The listing builds one solid part. Answer for the finished solid, in the listing's coordinates (mm). Face numbers are marked on the shaded views. Give positions to 0.01 mm unless a question says otherwise; leave off trailing zeros. Write each loop counter-clockwise with the first axis right and the second up, starting at its lowest first coordinate (ties: lowest second). Pieces come first, ordered by that corner, then holes. Notation, with made-up numbers: (53.25, 28) - (74.25, 28) arc R36 cw to (74.25, 67) - close; hole circle Ø1 at (74, 71). An arc over 180 degrees is marked (long way). Answer as CSV lines item,"result". Start each with the question number.
(1) Find section D-D (y = -4.25). Write down the section's boundary in (x, z).
(2) Straight lines are drawn through the part: probe 1 along Y at (x, z) = (3.25, 12); probe 2 along Y at (x, z) = (3.25, 37); probe 3 along Y at (x, z) = (19.75, 35.5). For each, find the intervals that lie inside material, in ascending order.
(3) Find section B-B (z = 38.5). Write down the section's boundary in (x, y).
(4) Each of these flat-tipped pins is pushed along its axis until it touches: pin 1 Ø3 at (x, z) = (19, 37.5) entering from -Y; pin 2 Ø3 at (x, y) = (8.5, -3) entering from -Z; pin 3 Ø8 at (x, z) = (9, 4) entering from -Y. Where does it stop, or does it pass through?
(5) For a pull along Y with two mould halves and no side action, classify the marked faces 1, 2 and 3 as pulls with the +Y half, pulls with the -Y half, needs draft (parallel to the pull), parting line crosses it, or undercut.
(6) Find section C-C (z = 9). Write down the section's boundary in (x, y), then the cut area to 3 significant figures.
from build123d import *

# Parameters (mm, degrees)
F0_W     = 27
F0_H     = 43
F1_DEPTH = 2
F3_DEPTH = 27
F4_R     = 70
F5_R     = 0.5
F6_R     = 10
F7_R     = 0.99999
F8_R     = 0.2


# Not quite as in the source:
# - a fillet or chamfer is up to 0.001 mm smaller than in the source, because OpenCascade refuses the exact size


with BuildPart() as f1:
    # F0 (on Front) → F1 (new body)
    with BuildSketch(Plane.XZ):
        with Locations((13.5, 21.5)):
            Rectangle(F0_W, F0_H)
    extrude(amount=F1_DEPTH)

    # F2 (on Right) → F3 (join, through all)
    with BuildSketch(Plane.YZ):
        Polygon((0, 17.9200492635), (0, 23.7676580638), (-7, 43), (-7, 37.1523911997), align=None)
    extrude(amount=F3_DEPTH)

    # F4
    f4_edges = [f1.edges().sort_by_distance(p)[0] for p in [
        (13.5, -2, 23.415004),
    ]]
    fillet(f4_edges, radius=F4_R)

    # F5
    f5_edges = [f1.edges().sort_by_distance(p)[0] for p in [
        (13.5, -2, 29.262613),
    ]]
    fillet(f5_edges, radius=F5_R)

    # F6
    f6_edges = [f1.edges().sort_by_distance(p)[0] for p in [
        (13.5, -7, 37.152391),
    ]]
    fillet(f6_edges, radius=F6_R)

    # F7 (radius 1 in the source; OpenCascade refuses exactly that, so slightly less here)
    f7_edges = [f1.edges().sort_by_distance(p)[0] for p in [
        (13.5, -2, 43),
        (13.5, 0, 43),
        (13.5, -2, 0),
        (13.5, 0, 0),
    ]]
    fillet(f7_edges, radius=F7_R)

    # F8
    f8_edges = [f1.edges().sort_by_distance(p)[0] for p in [
        (13.5, -7, 43),
    ]]
    fillet(f8_edges, radius=F8_R)


solid = f1.part
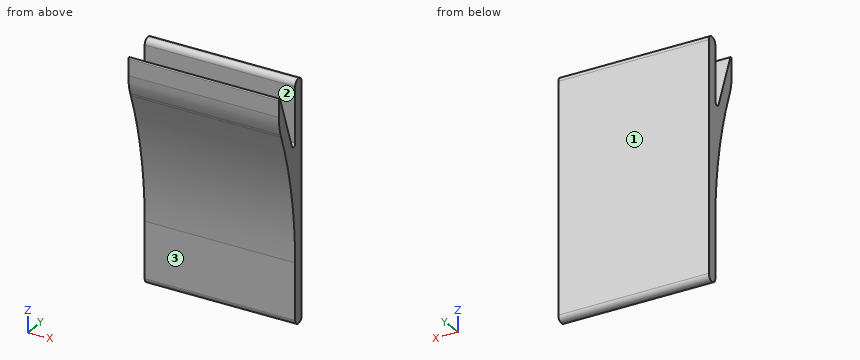
Result set:
1,outline,"(0, 28.68) - (27, 28.68) - (27, 35.44) - (0, 35.44) - close"
2,probe 1,"-2.01 to 0"
2,probe 2,"-6.81 to -4.82, -2 to 0"
2,probe 3,"-6.4 to -4.27, -2 to 0"
3,outline,"(0, -6.99) - (27, -6.99) - (27, -5.36) - (0, -5.36) - close; (0, -2) - (27, -2) - (27, 0) - (0, 0) - close"
4,pin 1,"y = -7"
4,pin 2,"z = 0.13"
4,pin 3,"y = -2"
5,face 1,"pulls with the +Y half"
5,face 2,"undercut"
5,face 3,"pulls with the -Y half"
6,outline,"(0, -2) - (27, -2) - (27, 0) - (0, 0) - close"
6,area,"54.0 mm^2"
